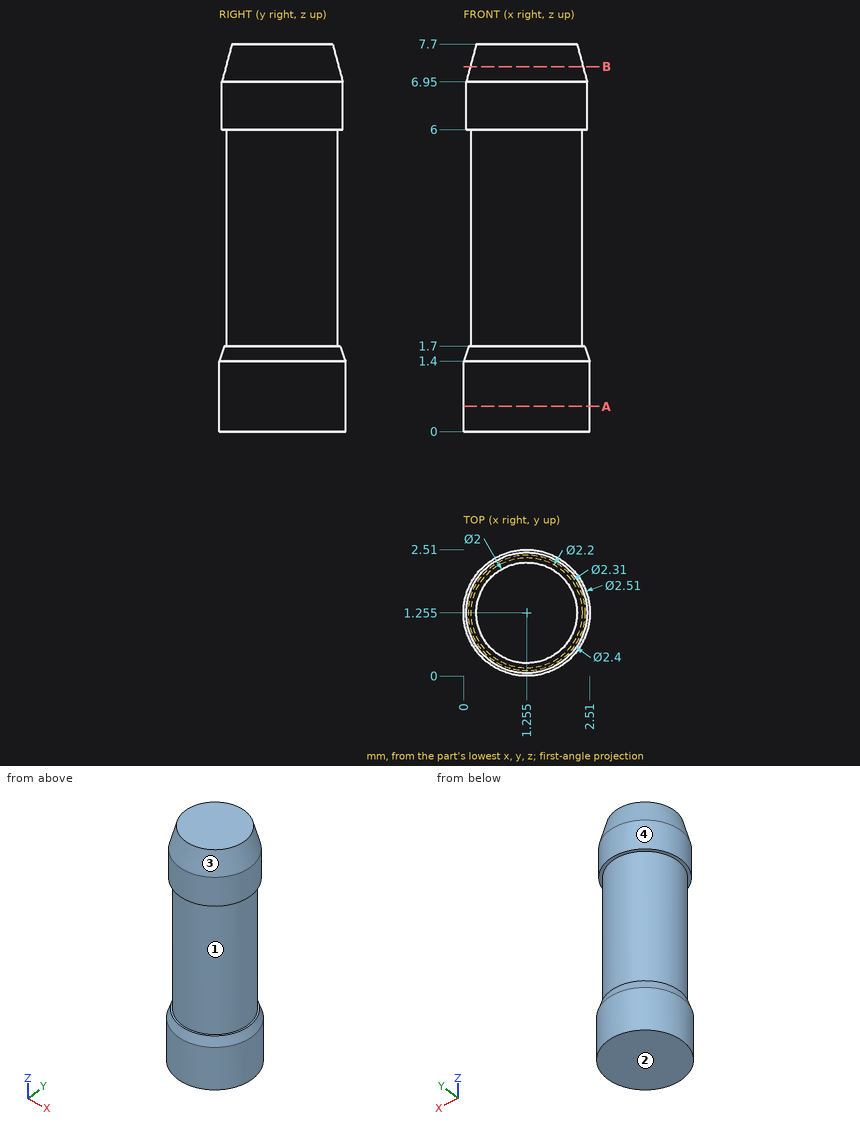
Could you check a few things on this drawing? It's one solid part, dimensions in mm from its lowest x, y, z. Round coordinates to 2 decimals unless told otherwise and drop trailing zeros. Order: outer loops, then holes, each group sorted by start corner. A loop starts at its lowest first (then second) coordinate and runs counter-clockwise, first axis right, second up.
(1) Imagine slicing it at A-A (z = 0.5). Write out the boundary of the cut face in (x, y) (3 decimals), plus the area to 3 significant figures.
Response values:
outline: circle Ø2.51 at (1.255, 1.255)
area: 4.95 mm2
(2) I'm going to push flat-ended pins straight in: pin 1 (1.5 mm diameter, centred on y = 1, z = 4, fed in from +X) (3 decimals); pin 2 (1.5 mm diameter, centred on x = 1.5, z = 2, fed in from +Y); pin 3 (1 mm diameter, centred on x = 0.5, z = 2.5, fed in from -Y); pin 4 (1.5 mm diameter, centred on x = 2, z = 3.5, fed in from +Y) (3 decimals). Where does each tip first touch, or does it pass through?
Response values:
pin 1: stops at x = 2.355
pin 2: stops at y = 2.51
pin 3: stops at y = 0.18
pin 4: stops at y = 2.355
(3) If we mould it in two halves opening along Z, with no side actions, what happens to the marked faces 1, 2, 3 and 4? For each: released by +Z, released by -Z, zero draft, split by the parting line, or undercut.
Response values:
face 1: undercut
face 2: released by -Z
face 3: released by +Z
face 4: zero draft
(4) Please list where these lines run through material, in increasing order: line 1 along X through (y, z) = (0.65, 0.75); line 2 along Y through (x, z) = (0.8, 5.5); line 3 along Y through (x, z) = (0.65, 4.25).
Response values:
line 1: x = 0.16 to 2.35
line 2: y = 0.25 to 2.26
line 3: y = 0.34 to 2.17
(5) Imagine slicing it at B-B (z = 7.25). Write out the boundary of the cut face in (x, y) (3 decimals), plus the area to 3 significant figures.
Response values:
outline: circle Ø2.24 at (1.255, 1.255)
area: 3.94 mm2
